Model file for the job. Use its own axes, mm. A direction names the side the tool comes from. Coordinates: 2 decimals unless noted, no trailing zeros. Order: outer loops, then holes, each group sorted by start corner. A loop starts at its lowest first (then second) coordinate and runs counter-clockwise, first axis right, second up. Notation, with made-up numbers: (-18, -27) -> (6, -27) arc R16 ccw to (6, -4) -> close; hole circle Ø11 at (-20, 8). An arc over 180 degrees is marked (long way). Return JSON: item names as keys, results as strings. Group by question number.
1) Probe line 1 (Y direction, x = -1.5, z = 2.5); line 2 (X direction, y = 7, z = -0.25); line 3 (X direction, y = 8, z = -1). List the from-to ranges inside material, lowest first.
2) Which spindle directions (+Z, -Z, +X, -X, +Y, -Y) get a long thin tool onto all of the face, cutting with end or side? Do faces 1 (the cylindrical face through (-2.87, 12.85, 1.67)), 2 (the cylindrical face through (0, 5, -2)). Say none if no direction does.
3) Cut at A-A (y = 5.25). Write the cut outline in (x, z), and give its area (3 significant figures).
4) Flat gauge pin, fed straight in: pin 1 (2 mm diameter, centred on y = 7.5, z = 2, fed in from +X). Where does the tip first touch, or does it go through?
from build123d import *

# Parameters (mm, degrees)
F0_R     = 2
F1_DEPTH = 10
F3_DEPTH = 3
F4_R     = 0.5


with BuildPart() as f1:
    # F0 (on Front) → F1 (new body)
    with BuildSketch(Plane.XZ):
        Circle(F0_R)
    extrude(amount=-F1_DEPTH)

    # F2 (on face) → F3 (join)
    with BuildSketch(Plane(origin=(0, 10, 0), x_dir=(-1, 0, 0), z_dir=(0, 1, 0))):
        Polygon((3.99994, -0.021899), (2.018935, 3.4531), (-1.981005, 3.474999), (-3.99994, 0.021899), (-2.018935, -3.4531), (1.981005, -3.474999), align=None)
    extrude(amount=F3_DEPTH)

    # F4
    f4_edges = [f1.edges().sort_by_distance(p)[0] for p in [
        (-2.990473, 13, -1.748449),
        (-3.009437, 13, 1.715601),
        (-0.018965, 13, 3.46405),
        (2.990473, 13, 1.748449),
        (3.009437, 13, -1.715601),
        (0.018965, 13, -3.46405),
    ]]
    fillet(f4_edges, radius=F4_R)


solid = f1.part
Answers below:
{
 "1": {"line 1": "y = 10 to 13", "line 2": "x = -1.98 to 1.98", "line 3": "x = -1.73 to 1.73"},
 "2": {"face 1": "+Z, -X, +Y", "face 2": "-Y"},
 "3": {"outline": "circle Ø4 at (0, 0)", "area": "12.6 mm^2"},
 "4": {"pin 1": "stops at x = 1.73"}
}
